```python
from build123d import *

# Parameters (mm, degrees)
SKETCH1_R           = 60
BOSS_EXTRUDE2_DEPTH = 4.4
SKETCH2_R           = 20
CUT_EXTRUDE1_DEPTH  = 20.9
SKETCH3_R           = 48.468089367
BOSS_EXTRUDE3_DEPTH = 3.9
SKETCH4_R           = 60
BOSS_EXTRUDE4_DEPTH = 4.4
SKETCH5_R           = 20
SKETCH5_R_2         = 3
BOSS_EXTRUDE5_DEPTH = 4
SKETCH7_R           = 5
CUT_EXTRUDE4_DEPTH  = 16


with BuildPart() as part:
    # Sketch1 → Boss-Extrude2 (new body)
    with BuildSketch(Plane.XY):
        Circle(SKETCH1_R)
    extrude(amount=BOSS_EXTRUDE2_DEPTH)

    # Sketch2 → Cut-Extrude1 (cut)
    with BuildSketch(Plane.XY.offset(4.4)):
        Circle(SKETCH2_R)
    extrude(amount=-CUT_EXTRUDE1_DEPTH, mode=Mode.SUBTRACT)

    # Sketch3 → Boss-Extrude3 (add)
    with BuildSketch(Plane.XY.offset(4.4)):
        Circle(SKETCH3_R)
    extrude(amount=BOSS_EXTRUDE3_DEPTH)

    # Sketch4 → Boss-Extrude4 (add)
    with BuildSketch(Plane.XY.offset(8.3)):
        Circle(SKETCH4_R)
    extrude(amount=BOSS_EXTRUDE4_DEPTH)

    # Sketch5 → Boss-Extrude5 (add)
    with BuildSketch(Plane(origin=(0, 0, 4.4), x_dir=(-1, 0, 0), z_dir=(0, 0, -1))):
        with Locations(Location((0, 0, 0), (0, 0, 180))):
            Circle(SKETCH5_R)
        Circle(SKETCH5_R_2, mode=Mode.SUBTRACT)
    extrude(amount=BOSS_EXTRUDE5_DEPTH)

    # Sketch7 → Cut-Extrude4 (cut)
    with BuildSketch(Plane(origin=(0, 0, 4.4), x_dir=(-1, 0, 0), z_dir=(0, 0, -1))):
        Circle(SKETCH7_R)
    extrude(amount=-CUT_EXTRUDE4_DEPTH, mode=Mode.SUBTRACT)


solid = part.part
```
Verification items for the finished model (mm, model axes). A direction names the side the tool comes from. Give positions to 0.01 mm unless a question says otherwise; leave off trailing zeros. Loops run counter-clockwise (first coordinate to the right, second up) from the corner with the lowest first, then second, coordinate; pieces in that order, holes last.
1. Mould release check, pull along Y, two halves, no side actions. Record for faces 1 (the flat face through (4, 0, 0.4)), 2 (the cylindrical face through (-59.94, 2.64, 10.47)), 3 (the flat face through (12, 1, 12.7)): released by +Y, released by -Y, zero draft, split by the parting line, or undercut.
2. Go/stop test with flat-tipped pins: pin 1 Ø1 at (x, z) = (-38, 10.5) entering from -Y; pin 2 Ø1.5 at (x, z) = (-47.5, 11) entering from +Y; pin 3 Ø7 at (x, y) = (0, 0) entering from +Z. Record where each tip stops, or that it passes through.
3. Section check D-D, the plane x = -24. Enter the section's corners in (y, z), then the cut area to 3 significant figures.
4. Set-up check for faces 4 (the flat face through (49, 0, 8.3)), 5 (the cylindrical face through (1.08, -4.88, 8.49)), 6 (the cylindrical face through (-4.336, -19.524, 0.203)): record each of +Z, -Z, +X, -X, +Y, -Y from which the full face is reachable in a straight line by a thin tool's end or side.
5. Section check C-C, the plane z = 10.5. Enter the section's corners in (x, y), then the cut area to 3 significant figures.
6. Section check A-A, the plane y = 0. Enter the section's corners in (x, z).
7. Thickness scan on line 1 (Z direction, x = 40, y = 37); line 2 (Y direction, x = 0, z = 0.25); line 3 (Y direction, x = 0, z = 2.9). Record the ranges inside material, lowest first.
Geometry says:
1. face 1: undercut
1. face 2: split by the parting line
1. face 3: zero draft
2. pin 1: stops at y = -46.84
2. pin 2: stops at y = 37.61
2. pin 3: stops at z = 4.4
3. outline: (-54.99, 0) - (54.99, 0) - (54.99, 4.4) - (42.11, 4.4) - (42.11, 8.3) - (54.99, 8.3) - (54.99, 12.7) - (-54.99, 12.7) - (-54.99, 8.3) - (-42.11, 8.3) - (-42.11, 4.4) - (-54.99, 4.4) - close
3. area: 1,300 mm2
4. face 4: none
4. face 5: +Z
4. face 6: -Z
5. outline: circle Ø120 at (0, 0); hole circle Ø10 at (0, 0)
5. area: 11,200 mm2
6. outline: (-60, 0) - (-20, 0) - (-20, 0.4) - (-3, 0.4) - (-3, 4.4) - (-5, 4.4) - (-5, 12.7) - (-60, 12.7) - (-60, 8.3) - (-48.47, 8.3) - (-48.47, 4.4) - (-60, 4.4) - close; (3, 0.4) - (20, 0.4) - (20, 0) - (60, 0) - (60, 4.4) - (48.47, 4.4) - (48.47, 8.3) - (60, 8.3) - (60, 12.7) - (5, 12.7) - (5, 4.4) - (3, 4.4) - close
7. line 1: z = 0 to 4.4, 8.3 to 12.7
7. line 2: y = -60 to -20, 20 to 60
7. line 3: y = -60 to -3, 3 to 60
